Design review of the part built by this model. Coordinates are the model's own, in mm. Face numbers are marked on the shaded views. Give positions to 0.01 mm unless a question says otherwise; leave off trailing zeros. Loops run counter-clockwise (first coordinate to the right, second up) from the corner with the lowest first, then second, coordinate; pieces in that order, holes last.
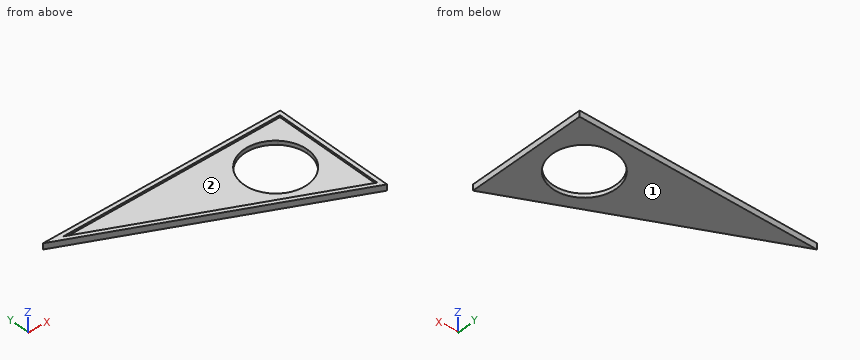
from build123d import *

# Parameters (mm, degrees)
F1_DEPTH = 3
F2_T     = -2
F4_DEPTH = 2.001


# Not quite as in the source:
# - ends of sketch curves that miss each other by under 0.0002 mm in the source are joined


with BuildPart() as f1:
    # F0 (on Top) → F1 (new body)
    with BuildSketch(Plane.XY):
        Polygon((0, -60), (0, 0), (-120, 0), align=None)
    extrude(amount=F1_DEPTH)

    # F2
    f2_openings = [f1.faces().sort_by_distance(p)[0] for p in [
        (-40, -20, 3),
    ]]
    offset(amount=F2_T, openings=f2_openings)

    # F3 (on face) → F4 (cut, through all)
    with BuildSketch(Plane.XY.offset(2)):
        with BuildLine():
            ThreePointArc((-12.0208152802, -12.0208152802), (-38.1165962993, -29.457458697), (-7.3345237792, -23.3345237792))
            ThreePointArc((-7.3345237792, -23.3345237792), (-8.552451259, -17.2115888613), (-12.0208152802, -12.0208152802))
        make_face()
    extrude(amount=-F4_DEPTH, mode=Mode.SUBTRACT)


solid = f1.part
Q1. Take a section at A-A (z = 0.9). Give the boundary of the cut face in (x, y), plus the area to 3 significant figures.
Results:
outline: (-120, 0) - (0, -60) - (0, 0) - close; hole circle Ø32 at (-23.33, -23.33)
area: 2,800 mm2
Q2. Insertion check: pin 1 (0.8 mm diameter, centred on y = -24, z = 2.5, fed in from -X); pin 2 (0.8 mm diameter, centred on x = -44, z = 2.5, fed in from -Y); pin 3 (8 mm diameter, centred on x = -43.5, y = -31, fed in from +Z). Each pin has a flat end and moves straight along its axis. Give the tip position at first contact, or say it passes through.
Results:
pin 1: stops at x = -72.8
pin 2: stops at y = -38.2
pin 3: stops at z = 2
Q3. Take a section at C-C (x = -101.5). Give the boundary of the cut face in (y, z), plus the area to 3 significant figures.
Results:
outline: (-9.25, 0) - (0, 0) - (0, 3) - (-2, 3) - (-2, 2) - (-7.01, 2) - (-7.01, 3) - (-9.25, 3) - close
area: 22.7 mm2
Q4. Take a section at B-B (y = -35.5). Give the boundary of the cut face in (x, z).
Results:
outline: (-49, 0) - (-33.73, 0) - (-33.73, 2) - (-44.53, 2) - (-44.53, 3) - (-49, 3) - close; (-12.94, 0) - (0, 0) - (0, 3) - (-2, 3) - (-2, 2) - (-12.94, 2) - close
Q5. Wall thickness on line 1 (Z direction, x = -91.5, y = -11); line 2 (X direction, y = -43.5, z = 2.8); line 3 (Y direction, x = -4.5, z = 2.65): over which ranges is each line inside the solid? List them lowest first.
Results:
line 1: z = 0 to 2
line 2: x = -33 to -28.53, -2 to 0
line 3: y = -57.75 to -55.51, -2 to 0
Q6. Draft analysis for pull direction Y (two halves, no side actions). For the marked faces 1 and 2, state which applies: pulls with the +Y half, pulls with the -Y half, needs draft (parallel to the pull), parting line crosses it, or undercut.
Results:
face 1: needs draft
face 2: undercut
Q7. Take a section at D-D (y = -4). Give the boundary of the cut face in (x, z), plus the area to 3 significant figures.
Results:
outline: (-112, 0) - (0, 0) - (0, 3) - (-2, 3) - (-2, 2) - (-107.53, 2) - (-107.53, 3) - (-112, 3) - close
area: 230 mm2
